```python
from build123d import *

# Parameters (mm, degrees)
F0_W     = 37
F0_H     = 34
F0_R     = 1
F0_R_2   = 4.8
F1_DEPTH = 4
F0_R_3   = 3.75
F2_DEPTH = 13
F3_SIZE  = 0.75
F0_R_4   = 1.25
F4_DEPTH = 2


with BuildPart() as f1:
    # F0 (on Top) → F1 (new body)
    with BuildSketch(Plane.XY):
        with Locations((-1.5, 0)):
            Rectangle(F0_W, F0_H)
        Polygon((-19.25, -15.510363), (-19.25, -13.489637), (-17.5, -12.479274), (-15.75, -13.489637), (-15.75, -15.510363), (-17.5, -16.520726), align=None, mode=Mode.SUBTRACT)
        with Locations((-8.5, -8.5)):
            Circle(F0_R, mode=Mode.SUBTRACT)
        Polygon((14.5, -16.520726), (12.75, -15.510363), (12.75, -13.489637), (14.5, -12.479274), (16.25, -13.489637), (16.25, -15.510363), align=None, mode=Mode.SUBTRACT)
        with Locations((8.5, -8.5)):
            Circle(F0_R, mode=Mode.SUBTRACT)
        Polygon((-19.25, 15.510363), (-17.5, 16.520726), (-15.75, 15.510363), (-15.75, 13.489637), (-17.5, 12.479274), (-19.25, 13.489637), align=None, mode=Mode.SUBTRACT)
        with Locations((-8.5, 8.5)):
            Circle(F0_R, mode=Mode.SUBTRACT)
        Circle(F0_R_2, mode=Mode.SUBTRACT)
        with Locations((8.5, 8.5)):
            Circle(F0_R, mode=Mode.SUBTRACT)
        Polygon((14.5, 12.479274), (12.75, 13.489637), (12.75, 15.510363), (14.5, 16.520726), (16.25, 15.510363), (16.25, 13.489637), align=None, mode=Mode.SUBTRACT)
    extrude(amount=F1_DEPTH)

    # F0 (on Top) → F2 (join)
    with BuildSketch(Plane.XY):
        Circle(F0_R_2)
        Circle(F0_R_3, mode=Mode.SUBTRACT)
    extrude(amount=F2_DEPTH)

    # F3
    f3_edges = [f1.edges().sort_by_distance(p)[0] for p in [
        (-4.8, 0, 13),
    ]]
    chamfer(f3_edges, length=F3_SIZE)

    # F0 (on Top) → F4 (join)
    with BuildSketch(Plane.XY):
        Polygon((-17.5, -12.479274), (-19.25, -13.489637), (-19.25, -15.510363), (-17.5, -16.520726), (-15.75, -15.510363), (-15.75, -13.489637), align=None)
        with Locations((-17.5, -14.5)):
            Circle(F0_R_4, mode=Mode.SUBTRACT)
        Polygon((12.75, -13.489637), (12.75, -15.510363), (14.5, -16.520726), (16.25, -15.510363), (16.25, -13.489637), (14.5, -12.479274), align=None)
        with Locations((14.5, -14.5)):
            Circle(F0_R_4, mode=Mode.SUBTRACT)
        Polygon((12.75, 15.510363), (12.75, 13.489637), (14.5, 12.479274), (16.25, 13.489637), (16.25, 15.510363), (14.5, 16.520726), align=None)
        with Locations((14.5, 14.5)):
            Circle(F0_R_4, mode=Mode.SUBTRACT)
        Polygon((-15.75, 15.510363), (-17.5, 16.520726), (-19.25, 15.510363), (-19.25, 13.489637), (-17.5, 12.479274), (-15.75, 13.489637), align=None)
        with Locations((-17.5, 14.5)):
            Circle(F0_R_4, mode=Mode.SUBTRACT)
    extrude(amount=F4_DEPTH)


solid = f1.part
```
Could you check a few things on this model? Use its own coordinates, in mm. A direction names the side the tool comes from. Round coordinates to 2 decimals unless told otherwise and drop trailing zeros. Loops run counter-clockwise (first coordinate to the right, second up) from the corner with the lowest first, then second, coordinate; pieces in that order, holes last.
Q1. Thinking about a two-plate mould opening in X: for faces 1 (the flat face through (-6, 0, 4)), 2 (the flat face through (13, 14, 2)), which applies, pulls with the +X half, pulls with the -X half, needs draft (parallel to the pull), parting line crosses it, or undercut?
Q2. I want a section at A-A (y = 14.5). Write out the boundary of the cut face in (x, z).
Q3. On a 3-axis mill with a long thin cutter (end or side, diameter ignored), from which of +Z, -Z, +X, -X, +Y, -Y can I reach the whole of each face in a straight line? I mean faces 3 (the cylindrical face through (14.34, -13.26, 0.99)), 4 (the flat face through (-15.75, 15, 3)). Say none if no direction works.
Q4. I want a section at D-D (x = 0). Write out the boundary of the cut face in (y, z), and give its area (3 significant figures).
Q5. For P1, Ø3, axis at x = 8.5, y = -8.5, coming from the +Z side; P2, Ø10, axis at x = 1, y = -4, coming from the +Z side; P3, Ø3, axis at x = 14.5, y = -14.5, coming from the +Z side; P4, Ø1.5, axis at x = -3.5, z = 9.5, coming from the +Y side, each with a flat end and sliding along its axis, tell me the tip position at first contact or that it passes through.
Q6. Please list where these lines run through material, in increasing order: L1, parallel to Y at x = -8.5, z = 2; L2, parallel to Y at x = 14.5, z = 0.95; L3, parallel to Z at x = -6, y = 1.
Q7. I want a section at B-B (x = 8.5). Write out the boundary of the cut face in (y, z).
Q8. I want a section at C-C (y = 0). Write out the boundary of the cut face in (x, z).
Answer below:
1. face 1: needs draft
1. face 2: undercut
2. outline: (-20, 0) - (-18.75, 0) - (-18.75, 2) - (-19.25, 2) - (-19.25, 4) - (-20, 4) - close; (-16.25, 0) - (13.25, 0) - (13.25, 2) - (12.75, 2) - (12.75, 4) - (-15.75, 4) - (-15.75, 2) - (-16.25, 2) - close; (15.75, 0) - (17, 0) - (17, 4) - (16.25, 4) - (16.25, 2) - (15.75, 2) - close
3. face 3: +Z, -Z
3. face 4: +Z
4. outline: (-17, 0) - (-3.75, 0) - (-3.75, 13) - (-4.05, 13) - (-4.8, 12.25) - (-4.8, 4) - (-17, 4) - close; (3.75, 0) - (17, 0) - (17, 4) - (4.8, 4) - (4.8, 12.25) - (4.05, 13) - (3.75, 13) - close
4. area: 124 mm2
5. P1: stops at z = 4
5. P2: stops at z = 13
5. P3: stops at z = 2
5. P4: stops at y = 3.93
6. L1: y = -17 to -9.5, -7.5 to 7.5, 9.5 to 17
6. L2: y = -17 to -15.75, -13.25 to 13.25, 15.75 to 17
6. L3: z = 0 to 4
7. outline: (-17, 0) - (-9.5, 0) - (-9.5, 4) - (-17, 4) - close; (-7.5, 0) - (7.5, 0) - (7.5, 4) - (-7.5, 4) - close; (9.5, 0) - (17, 0) - (17, 4) - (9.5, 4) - close
8. outline: (-20, 0) - (-3.75, 0) - (-3.75, 13) - (-4.05, 13) - (-4.8, 12.25) - (-4.8, 4) - (-20, 4) - close; (3.75, 0) - (17, 0) - (17, 4) - (4.8, 4) - (4.8, 12.25) - (4.05, 13) - (3.75, 13) - close
